Geometry: final body of the model. Coordinates: model frame, mm. A direction names the side the tool comes from. Give positions to 0.01 mm unless a question says otherwise; leave off trailing zeros. Write each loop counter-clockwise with the first axis right and the second up, starting at its lowest first coordinate (ties: lowest second). Pieces come first, ordered by that corner, then holes. Notation, with made-up numbers: M 5,2.5 L 60,2.5 A24 cw 60,25.5 Z; hole C -28,63.25 d10. An arc over 180 degrees is marked long. Use a Markdown table: item, result. Add a question column.
1) Set-up query: faces 3 (the flat face through (-8, -12, 18)), 4 (the flat face through (-2.36, -9.98, 20.03)). Return all of +Z, -Z, +X, -X, +Y, -Y with unobstructed straight access to the full face (end or side cutting, diameter ignored); none if empty.
2) Pin query (flat end, axial travel): pin 1 (10 mm diameter, centred on x = 1.5, y = -18, fed in from +Z); pin 2 (5 mm diameter, centred on x = 8, y = 16.5, fed in from -Z); pin 3 (1.5 mm diameter, centred on y = -10.5, z = 18.5, fed in from +X). Return the tip coordinate at first contact, or that it passes through.
3) Line query: line 1 (Y direction, x = -0.5, z = 2); line 2 (X direction, y = -21.5, z = 21.75); line 3 (Y direction, x = -2, z = 16). Output: solid intervals per line, ascending.
4) Section C-C on y = -10. Return the cut outline in (x, z), then the cut area to 3 significant figures.
5) Draft query along X for faces 1 (the flat face through (7.506, 7.09, 20.028)), 2 (the cylindrical face through (6.94, 31.24, 12.82)). Return one class per face: +X half, -X half, draft (parallel to the pull), parting line (faces both ways), or undercut.
6) Section D-D on x = -13.5. Return the cut outline in (y, z), then the cut area to 3 significant figures.
7) Section A-A on z = 16. Return the cut outline in (x, y), then the cut area to 3 significant figures.
8) Section B-B on x = 0. Return the cut outline in (y, z), then the cut area to 3 significant figures.
```python
from build123d import *
from build123d.topology import SkipClean

# Parameters (mm, degrees)
ESQUISSE1_R                  = 32
BOSS_EXTRU_1_DEPTH           = 26
ESQUISSE3_R                  = 23.25
ENL_V_MAT_EXTRU_2_DEPTH      = 4
ENL_V_START                  = -18
ESQUISSE4_R                  = 23.25
ENL_V_MAT_EXTRU_3_DEPTH      = 18
ESQUISSE6_R                  = 8
BOSS_EXTRU_5_DEPTH           = 3
ESQUISSE2_R                  = 2
ENL_V_MAT_EXTRU_4_DEPTH      = 53.191953403
ENL_V_MAT_EXTRU_5_DEPTH      = 3
ENL_V_MAT_EXTRU_8_DEPTH      = 51.318982502
R_P_TITION_CIRCULAIRE1_COUNT = 6
ENL_V_MAT_EXTRU_9_DEPTH      = 51.318982502
R_P_TITION_CIRCULAIRE2_COUNT = 6


with BuildPart() as part:
    # Esquisse1 → Boss.-Extru.1 (new body)
    with BuildSketch(Plane.XY):
        with Locations(Location((0, 0, 0), (0, 0, 180))):
            Circle(ESQUISSE1_R)
    extrude(amount=BOSS_EXTRU_1_DEPTH)

    # Esquisse3 → Enlèv. mat.-Extru.2 (cut)
    with BuildSketch(Plane.XY.offset(26)):
        Circle(ESQUISSE3_R)
    extrude(amount=-ENL_V_MAT_EXTRU_2_DEPTH, mode=Mode.SUBTRACT)

    # Esquisse4 → Enlèv. mat.-Extru.3 (cut)
    with BuildSketch(Plane(origin=(0, 0, 0), x_dir=(-1, 0, 0), z_dir=(0, 0, -1)).offset(ENL_V_START)):
        with Locations(Location((0, 0, 0), (0, 0, 180))):
            Circle(ESQUISSE4_R)
    extrude(amount=ENL_V_MAT_EXTRU_3_DEPTH, mode=Mode.SUBTRACT)

    # Esquisse6 → Boss.-Extru.5 (add)
    with BuildSketch(Plane(origin=(0, 0, 18), x_dir=(-1, 0, 0), z_dir=(0, 0, -1))):
        Circle(ESQUISSE6_R)
    extrude(amount=BOSS_EXTRU_5_DEPTH)

    # Esquisse2 → Enlèv. mat.-Extru.4 (cut, through all)
    with BuildSketch(Plane.XY.offset(26)):
        Circle(ESQUISSE2_R)
    extrude(amount=-ENL_V_MAT_EXTRU_4_DEPTH, mode=Mode.SUBTRACT)

    # Esquisse7 → Enlèv. mat.-Extru.5 (cut)
    with BuildSketch(Plane(origin=(0, 0, 15), x_dir=(-1, 0, 0), z_dir=(0, 0, -1))):
        Polygon((-3.464101615, 6), (3.464101615, 6), (6.92820323, 0), (3.464101615, -6), (-3.464101615, -6), (-6.92820323, 0), align=None)
    extrude(amount=-ENL_V_MAT_EXTRU_5_DEPTH, mode=Mode.SUBTRACT)

    # Esquisse8 → Enlèv. mat.-Extru.8 (cut, through all)
    with BuildSketch(Plane.XY.offset(22)):
        with BuildLine():
            Line((-3.25, 12.171773317), (-1.5, 7.858116823))
            ThreePointArc((-1.5, 7.858116823), (0, 8), (1.5, 7.858116823))
            Line((1.5, 7.858116823), (3.25, 12.171773317))
            Line((3.25, 12.171773317), (2.75, 23.086792761))
            ThreePointArc((2.75, 23.086792761), (0, 23.25), (-2.75, 23.086792761))
            Line((-2.75, 23.086792761), (-3.25, 12.171773317))
        make_face()
    enl_v_mat_extru_8 = extrude(amount=-ENL_V_MAT_EXTRU_8_DEPTH, mode=Mode.SUBTRACT)

    # Répétition circulaire1: Enlèv. mat.-Extru.8 ×6 about axis
    with SkipClean():  # the faces are left unmerged after this step: merging them gives an invalid solid
        r_p_tition_circulaire1_axis = Axis((0, 0, 0), (0, 0, 1))
        for i in range(1, R_P_TITION_CIRCULAIRE1_COUNT):
            add(enl_v_mat_extru_8.rotate(r_p_tition_circulaire1_axis, i * 360 / R_P_TITION_CIRCULAIRE1_COUNT), mode=Mode.SUBTRACT)
    add(part.part.scale(1), mode=Mode.REPLACE)  # the faces are merged on a copy

    # Esquisse9 → Enlèv. mat.-Extru.9 (cut, through all)
    with BuildSketch(Plane.XY.offset(22)):
        with BuildLine():
            Line((7.868982797, 13.031089676), (7.457138731, 22.021661653))
            ThreePointArc((7.457138731, 22.021661653), (12.01849939, 19.902717714), (16.017447426, 16.852414603))
            Line((16.017447426, 16.852414603), (7.868982797, 13.031089676))
        make_face()
    enl_v_mat_extru_9 = extrude(amount=-ENL_V_MAT_EXTRU_9_DEPTH, mode=Mode.SUBTRACT)

    # Répétition circulaire2: Enlèv. mat.-Extru.9 ×6 about axis
    r_p_tition_circulaire2_axis = Axis((0, 0, 0), (0, 0, 1))
    for i in range(1, R_P_TITION_CIRCULAIRE2_COUNT):
        add(enl_v_mat_extru_9.rotate(r_p_tition_circulaire2_axis, i * 360 / R_P_TITION_CIRCULAIRE2_COUNT), mode=Mode.SUBTRACT)


solid = part.part
```
Found:
| question | item | result |
|---|---|---|
| 1 | face 3 | -Z |
| 1 | face 4 | +Z, -Z |
| 2 | pin 1 | z = 22 |
| 2 | pin 2 | z = 18 |
| 2 | pin 3 | x = 30.48 |
| 3 | line 1 | -32 to -23.24, 23.24 to 32 |
| 3 | line 2 | -23.7 to -8.85, -7.48 to -2.82, 2.82 to 6.65, 8.85 to 23.7 |
| 3 | line 3 | -31.94 to -23.16, -7.75 to -6, 6 to 7.75, 23.16 to 31.94 |
| 4 | outline | M -30.4,0 L -20.99,0 L -20.99,26 L -30.4,26 Z; M -11.04,18 L -2.37,18 L -2.37,22 L -11.04,22 Z; M 2.37,18 L 11.04,18 L 11.04,22 L 2.37,22 Z; M 20.99,0 L 30.4,0 L 30.4,26 L 20.99,26 Z |
| 4 | area | 559 mm² |
| 5 | face 1 | undercut |
| 5 | face 2 | parting line |
| 6 | outline | M -29.01,0 L -18.93,0 L -18.93,26 L -29.01,26 Z; M -15.67,18 L -11.27,18 L -11.27,22 L -15.67,22 Z; M -4.13,18 L 4.13,18 L 4.13,22 L -4.13,22 Z; M 11.27,18 L 16.51,18 L 16.51,22 L 11.27,22 Z; M 18.93,0 L 29.01,0 L 29.01,26 L 18.93,26 Z |
| 6 | area | 596 mm² |
| 7 | outline | C 0,0 d64; C 0,0 d16; hole C 0,0 d46.5; hole M -6.93,0 L -3.46,-6 L 3.46,-6 L 6.93,0 L 3.46,6 L -3.46,6 Z |
| 7 | area | 1,600 mm² |
| 8 | outline | M -32,0 L -23.25,0 L -23.25,26 L -32,26 Z; M -8,15 L -6,15 L -6,18 L -2,18 L -2,22 L -8,22 Z; M 2,18 L 6,18 L 6,15 L 8,15 L 8,22 L 2,22 Z; M 23.25,0 L 32,0 L 32,26 L 23.25,26 Z |
| 8 | area | 515 mm² |
